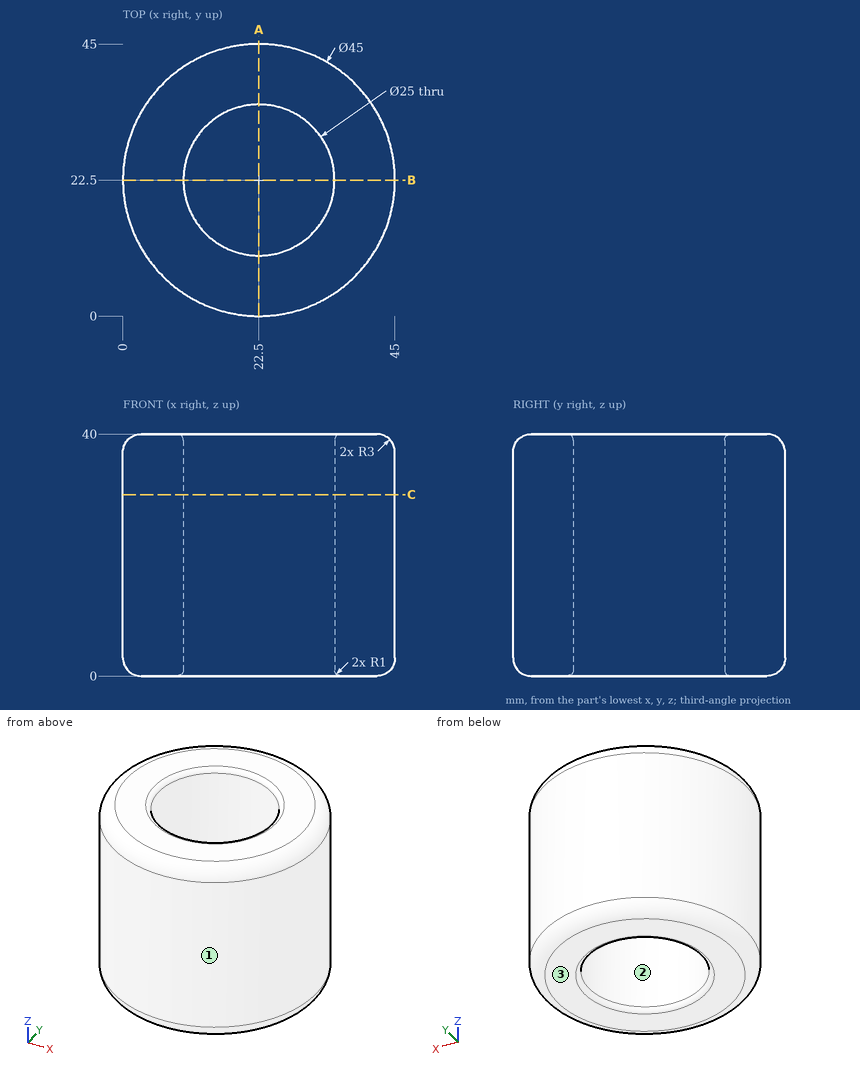
Study the drawing (mm; zero at the part's minimum x, y, z) and answer. Round coordinates to 2 decimals unless told otherwise and drop trailing zeros. Loops run counter-clockwise (first coordinate to the right, second up) from the corner with the lowest first, then second, coordinate; pieces in that order, holes last.
Q1. Given pin 1 Ø1.5 at (x, z) = (13.5, 25.5) entering from +Y; pin 2 Ø4 at (y, z) = (29.5, 33) entering from +X; pin 3 Ø2 at (x, z) = (25.5, 28) entering from +Y, each flat-ended and moving along its own axis, determine where each tip first touches the part or whether it passes through.
Q2. Find the intervals of material crossed by line 1 (Y direction, x = 22, z = 21); line 2 (X direction, y = 26, z = 26), in increasing order.
Q3. Section C-C, the plane z = 30 is taken. Determine the outline of the cut face in (x, y).
Q4. For a pull along Y with two mould halves and no side action, classify the marked faces 1, 2 and 3 as released by +Y, released by -Y, zero draft, split by the parting line, or undercut.
Q5. Section A-A, the plane x = 22.5 is taken. Determine the outline of the cut face in (y, z).
Completed:
1. pin 1: stops at y = 43.43
1. pin 2: stops at x = 44.44
1. pin 3: stops at y = 44.91
2. line 1: y = 0.01 to 10.01, 34.99 to 44.99
2. line 2: x = 0.27 to 10.5, 34.5 to 44.73
3. outline: circle Ø45 at (22.5, 22.5); hole circle Ø25 at (22.5, 22.5)
4. face 1: split by the parting line
4. face 2: undercut
4. face 3: zero draft
5. outline: (0, 3) arc R3 ccw to (3, 0) - (9, 0) arc R1 ccw to (10, 1) - (10, 39) arc R1 ccw to (9, 40) - (3, 40) arc R3 ccw to (0, 37) - close; (35, 1) arc R1 ccw to (36, 0) - (42, 0) arc R3 ccw to (45, 3) - (45, 37) arc R3 ccw to (42, 40) - (36, 40) arc R1 ccw to (35, 39) - close
